Could you check a few things on this drawing? It's one solid part, dimensions in mm from its lowest x, y, z. A direction names the side the tool comes from. Coordinates: 2 decimals unless noted, no trailing zeros. Loops run counter-clockwise (first coordinate to the right, second up) from the corner with the lowest first, then second, coordinate; pieces in that order, holes last. Notation, with made-up numbers: M 23.25,-35 L 82.25,-35 A29 cw 82.25,3 Z; hole C -17.75,56 d10. An arc over 180 degrees is marked long. Answer as a JSON object with one key per item and string values. Group by question number.
Item 1: Which directions (+Z, -Z, +X, -X, +Y, -Y) give clear straight access to the entire face, cutting with the end or side of a thin tool? Please do the marked faces 1 and 2.
Item 2: We'd pull the mould along Y, two halves only. Please class the marked faces 3, 4, 5 and 6: +Y half, -Y half, draft (parallel to the pull), parting line (faces both ways), or undercut.
Item 3: If I drill on line 1 (Y direction, x = 194, z = 13.5) (1 decimal); line 2 (X direction, y = 27.5, z = 9.75); line 3 (Y direction, x = 75, z = 10.5) (1 decimal), over which ranges is the centre line in solid material (lowest first)?
Item 4: Suppose I cut it at D-D (x = 162.5). Write out the boundary of the cut face in (y, z) (1 decimal).
Item 5: Suppose I cut it at A-A (y = 86.5). Write out the boundary of the cut face in (x, z), then the cut area to 3 significant figures.
Item 6: Suppose I cut it at C-C (x = 80). Write out the boundary of the cut face in (y, z) (1 decimal).
Item 7: I'm going to push flat-ended pins straight in: pin 1 Ø10 at (x, z) = (93, 11.5) entering from -Y; pin 2 Ø7.5 at (x, z) = (133, 14) entering from +Y; pin 3 Ø1 at (x, z) = (178.5, 12) entering from -Y (1 decimal). Where does each tip first touch, or does it pass through?
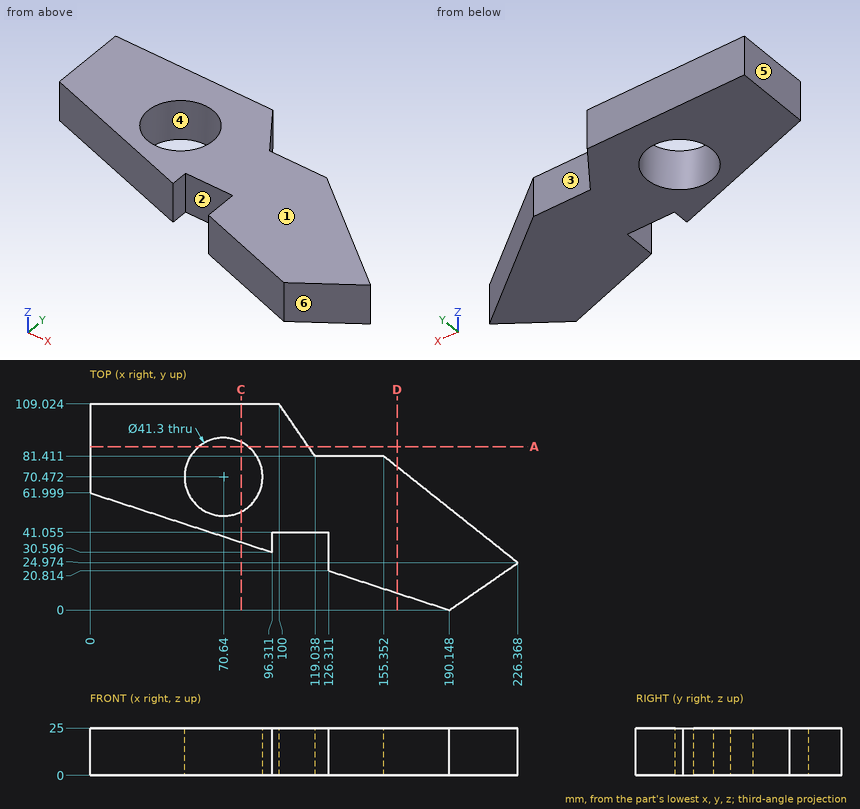
From the geometry:
{
 "1": {"face 1": "+Z, +X, -X, +Y, -Y", "face 2": "+Z, -Z, -Y"},
 "2": {"face 3": "+Y half", "face 4": "undercut", "face 5": "draft", "face 6": "-Y half"},
 "3": {"line 1": "2.7 to 50.7", "line 2": "126.31 to 223.19", "line 3": "37.5 to 50.3, 90.7 to 109"},
 "4": {"outline": "M 9,0 L 75.7,0 L 75.7,25 L 9,25 Z"},
 "5": {"outline": "M 0,0 L 57.62,0 L 57.62,25 L 0,25 Z; M 83.66,0 L 115.53,0 L 115.53,25 L 83.66,25 Z", "area": "2,240 mm2"},
 "6": {"outline": "M 35.9,0 L 52.1,0 L 52.1,25 L 35.9,25 Z; M 88.9,0 L 109,0 L 109,25 L 88.9,25 Z"},
 "7": {"pin 1": "y = 30.6", "pin 2": "y = 81.41", "pin 3": "y = 3.6"}
}
